The listing builds one solid part. Answer for the finished solid, in the listing's coordinates (mm). A direction names the side the tool comes from. Round coordinates to 2 decimals unless told otherwise and drop trailing zeros. Loops run counter-clockwise (first coordinate to the right, second up) from the corner with the lowest first, then second, coordinate; pieces in that order, holes last. Notation, with made-up numbers: (11.25, 73) -> (67.25, 73) arc R36 ccw to (67.25, 107) -> close; hole circle Ø7 at (-8.5, 16.25). An arc over 180 degrees is marked (long way). One line per question, with ' | ' between items.
from build123d import *

# Parameters (mm, degrees)
SKETCH1_R           = 42.5
BOSS_EXTRUDE1_DEPTH = 2.5
SKETCH3_W           = 13
SKETCH3_H           = 18
BOSS_EXTRUDE2_DEPTH = 20
SKETCH4_R           = 8.9
CUT_EXTRUDE2_DEPTH  = 20
SKETCH5_R           = 8.9
CUT_EXTRUDE3_DEPTH  = 20
SKETCH6_R           = 8.9
CUT_EXTRUDE4_DEPTH  = 20
CUT_EXTRUDE5_START  = -20
SKETCH7_R           = 8.9
CUT_EXTRUDE5_DEPTH  = 20
CUT_EXTRUDE6_START  = -20
SKETCH8_R           = 8.9
CUT_EXTRUDE6_DEPTH  = 20
CUT_EXTRUDE7_START  = -20
SKETCH9_R           = 8.9
CUT_EXTRUDE7_DEPTH  = 20
CUT_EXTRUDE8_DEPTH  = 76.388
SKETCH11_W          = 18
SKETCH11_H          = 4.285356177
CUT_EXTRUDE9_DEPTH  = 76.388
SKETCH12_R          = 18.204170311
CUT_EXTRUDE10_DEPTH = 76.388
SKETCH16_W          = 3.647311836
SKETCH16_H          = 1.511893876
CUT_EXTRUDE13_DEPTH = 101.6


with BuildPart() as part:
    # Sketch1 → Boss-Extrude1 (new body)
    with BuildSketch(Plane(origin=(0, 0, 0), x_dir=(1, 0, 0), z_dir=(0, 1, 0))):
        with Locations(Location((0, 0, 0), (0, 0, 270))):
            Circle(SKETCH1_R)
    extrude(amount=BOSS_EXTRUDE1_DEPTH)

    # Sketch3 → Boss-Extrude2 (add)
    with BuildSketch(Plane(origin=(0, 2.5, 0), x_dir=(1, 0, 0), z_dir=(0, 1, 0))):
        with Locations((-26.394376419, 0)):
            Rectangle(SKETCH3_W, SKETCH3_H)
        with Locations((26.394376419, 0)):
            Rectangle(SKETCH3_W, SKETCH3_H)
        Polygon((-8.599367677, 32.894541729), (-2.099367677, 21.63621148), (-17.687824945, 12.63621148), (-24.187824945, 23.894541729), align=None)
        Polygon((8.599367677, 32.894541729), (24.187824945, 23.894541729), (17.687824945, 12.63621148), (2.099367677, 21.63621148), align=None)
        Polygon((8.599367677, -32.894541729), (2.099367677, -21.63621148), (17.687824945, -12.63621148), (24.187824945, -23.894541729), align=None)
        Polygon((-8.599367677, -32.894541729), (-24.187824945, -23.894541729), (-17.687824945, -12.63621148), (-2.099367677, -21.63621148), align=None)
    extrude(amount=BOSS_EXTRUDE2_DEPTH)

    # Sketch4 → Cut-Extrude2 (cut)
    with BuildSketch(Plane.ZY.offset(32.894376419)):
        with Locations((0, 12.5)):
            Circle(SKETCH4_R)
    extrude(amount=-CUT_EXTRUDE2_DEPTH, mode=Mode.SUBTRACT)

    # Sketch5 → Cut-Extrude3 (cut)
    with BuildSketch(Plane(origin=(-16.393596311, 0, 28.394541729), x_dir=(0.8660254037844386, 0, 0.5000000000000003), z_dir=(-0.5000000000000003, 0, 0.8660254037844386))):
        with Locations((0, 12.5)):
            Circle(SKETCH5_R)
    extrude(amount=-CUT_EXTRUDE3_DEPTH, mode=Mode.SUBTRACT)

    # Sketch6 → Cut-Extrude4 (cut)
    with BuildSketch(Plane(origin=(16.393596311, 0, 28.394541729), x_dir=(0.8660254037844386, 0, -0.5000000000000003), z_dir=(0.5000000000000003, 0, 0.8660254037844386))):
        with Locations((0, 12.5)):
            Circle(SKETCH6_R)
    extrude(amount=-CUT_EXTRUDE4_DEPTH, mode=Mode.SUBTRACT)

    # Sketch7 → Cut-Extrude5 (cut)
    with BuildSketch(Plane(origin=(32.894376419, 0, 0), x_dir=(0, 0, -1), z_dir=(1, 0, 0)).offset(CUT_EXTRUDE5_START)):
        with Locations(Location((0, 12.5, 0), (0, 0, 180))):
            Circle(SKETCH7_R)
    extrude(amount=CUT_EXTRUDE5_DEPTH, mode=Mode.SUBTRACT)

    # Sketch8 → Cut-Extrude6 (cut)
    with BuildSketch(Plane(origin=(16.393596311, 0, -28.394541729), x_dir=(-0.8660254037844386, 0, -0.5000000000000003), z_dir=(0.5000000000000003, 0, -0.8660254037844386)).offset(CUT_EXTRUDE6_START)):
        with Locations(Location((0, 12.5, 0), (0, 0, 180))):
            Circle(SKETCH8_R)
    extrude(amount=CUT_EXTRUDE6_DEPTH, mode=Mode.SUBTRACT)

    # Sketch9 → Cut-Extrude7 (cut)
    with BuildSketch(Plane(origin=(-16.393596311, 0, -28.394541729), x_dir=(-0.8660254037844386, 0, 0.5000000000000003), z_dir=(-0.5000000000000003, 0, -0.8660254037844386)).offset(CUT_EXTRUDE7_START)):
        with Locations(Location((0, 12.5, 0), (0, 0, 180))):
            Circle(SKETCH9_R)
    extrude(amount=CUT_EXTRUDE7_DEPTH, mode=Mode.SUBTRACT)

    # Sketch10 → Cut-Extrude8 (cut)
    with BuildSketch(Plane(origin=(-16.393596311, 0, -28.394541729), x_dir=(-0.8660254037844386, 0, 0.5000000000000003), z_dir=(-0.5000000000000003, 0, -0.8660254037844386))):
        Polygon((-35.669118209, 18.214643823), (-9, 18.214643823), (-9, 22.5), (-6.822964603, 22.5), (-6.822964603, 25.559573076), (-35.669118209, 25.559573076), align=None)
        Polygon((-6.822964603, 25.559573076), (-6.822964603, 22.5), (9, 22.5), (9, 18.214643823), (33.747549551, 18.214643823), (33.747549551, 25.559573076), align=None)
    extrude(amount=-CUT_EXTRUDE8_DEPTH, mode=Mode.SUBTRACT)

    # Sketch11 → Cut-Extrude9 (cut)
    with BuildSketch(Plane(origin=(-16.393596311, 0, -28.394541729), x_dir=(-0.8660254037844386, 0, 0.5000000000000003), z_dir=(-0.5000000000000003, 0, -0.8660254037844386))):
        with Locations((0, 20.357321912)):
            Rectangle(SKETCH11_W, SKETCH11_H)
    extrude(amount=-CUT_EXTRUDE9_DEPTH, mode=Mode.SUBTRACT)

    # Sketch12 → Cut-Extrude10 (cut)
    with BuildSketch(Plane(origin=(0, 2.5, 0), x_dir=(1, 0, 0), z_dir=(0, 1, 0))):
        with Locations(Location((0, 0, 0), (0, 0, 270))):
            Circle(SKETCH12_R)
    extrude(amount=-CUT_EXTRUDE10_DEPTH, mode=Mode.SUBTRACT)

    # Sketch16 → Cut-Extrude13 (cut)
    with BuildSketch(Plane(origin=(0, 2.5, 0), x_dir=(1, 0, 0), z_dir=(0, 1, 0))):
        with Locations((0, -20.271174186)):
            Rectangle(SKETCH16_W, SKETCH16_H)
        with Locations((0, 20.271174186)):
            Rectangle(SKETCH16_W, SKETCH16_H)
    extrude(amount=-CUT_EXTRUDE13_DEPTH, mode=Mode.SUBTRACT)


solid = part.part
Q1. A cutting plane is placed at B-B on x = 0. Give the vertices of the cut face in (y, z).
Numbers:
outline: (0, -42.5) -> (2.5, -42.5) -> (2.5, -21.03) -> (0, -21.03) -> close; (0, -19.52) -> (2.5, -19.52) -> (2.5, -18.2) -> (0, -18.2) -> close; (0, 18.2) -> (2.5, 18.2) -> (2.5, 19.52) -> (0, 19.52) -> close; (0, 21.03) -> (2.5, 21.03) -> (2.5, 42.5) -> (0, 42.5) -> close
Q2. For a pull along Z with two mould halves and no side action, classify faces 1 (the face through (-15.275, 3.336, -29.04)), 2 (the face through (-26, 10, -9)), 3 (the face through (32.894, 3, -1)) as pulls with the +Z half, pulls with the -Z half, needs draft (parallel to the pull), parting line crosses it, or undercut.
Numbers:
face 1: pulls with the -Z half | face 2: undercut | face 3: needs draft
Q3. Given pin 1 Ø3 at (x, y) = (12.5, 9) entering from +Z; pin 2 Ø4 at (y, z) = (11.5, -27.5) entering from -X; pin 3 Ø4.5 at (y, z) = (7, -4.5) entering from -X; pin 4 Ø3 at (x, z) = (2.5, 31.5) entering from +Y, each flat-ended and moving along its own axis, determine where each tip first touches the part or whether it passes through.
Numbers:
pin 1: through | pin 2: x = -6.87 | pin 3: x = -32.89 | pin 4: y = 2.5
Q4. Find the intervals of material crossed by line 1 (X direction, y = 0.9, z = 0); line 2 (Z direction, x = -32, y = 14.75); line 3 (Y direction, x = 28, z = 0), in increasing order. Write a range as from..to.
Numbers:
line 1: -42.5..-18.2, 18.2..42.5 | line 2: -9..-8.61, 8.61..9 | line 3: 0..3.6
Q5. For faces 4 (the face through (0, 1, 21.027)), 5 (the face through (19.894, 3, -1)), 6 (the face through (5.304, 10.247, -27.187)), 7 (the face through (5.395, 10.247, 27.344)), 8 (the face through (-20.98, 10.25, 18.34)), determine the directions among +Z, -Z, +X, -X, +Y, -Y from which every point of the face is accessible in a straight line to the end or side of a thin tool.
Numbers:
face 4: +Y, -Y | face 5: +Y | face 6: -Z, +Y | face 7: +Z, +Y | face 8: -X, +Y
Q6. A cutting plane is placed at D-D on x = -36.5. Give the vertices of the cut face in (y, z), plus the area to 3 significant figures.
Numbers:
outline: (0, -21.77) -> (2.5, -21.77) -> (2.5, 21.77) -> (0, 21.77) -> close | area: 109 mm^2
Q7. A cutting plane is placed at A-A on z = 0. Give the vertices of the cut face in (x, y).
Numbers:
outline: (-42.5, 0) -> (-18.2, 0) -> (-18.2, 2.5) -> (-19.89, 2.5) -> (-19.89, 3.6) -> (-32.89, 3.6) -> (-32.89, 2.5) -> (-42.5, 2.5) -> close; (18.2, 0) -> (42.5, 0) -> (42.5, 2.5) -> (32.89, 2.5) -> (32.89, 3.6) -> (19.89, 3.6) -> (19.89, 2.5) -> (18.2, 2.5) -> close
